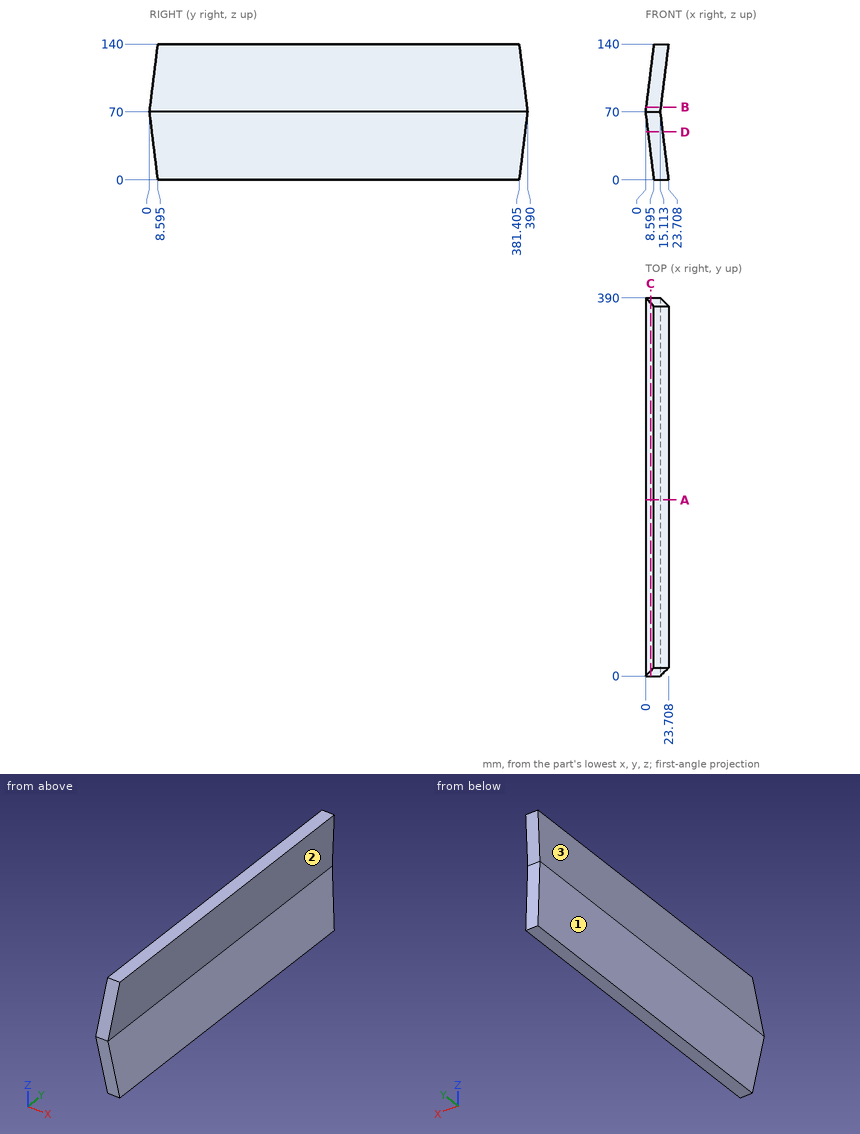
Input: dimensioned drawing with shaded views. Units: mm. Origin: part minimum x, y, z. Coordinates: 2 decimals unless noted, no trailing zeros. Loops run counter-clockwise (first coordinate to the right, second up) from the corner with the lowest first, then second, coordinate; pieces in that order, holes last. Notation, with made-up numbers: M 76.5,-10 L 112.5,-10 A28 cw 112.5,15 Z; hole C 72.5,87 d7. An arc over 180 degrees is marked long. One line per item, written item: value.
(1) Line query: line 1 along X through (y, z) = (51, 6.5); line 2 along X through (y, z) = (159.5, 59.5); line 3 along Y through (x, z) = (3, 87). Output: solid intervals per line, ascending. Write a range as from..to.
Filled in:
line 1: 7.8..22.91
line 2: 1.29..16.4
line 3: 2.09..387.91
(2) Section B-B (z = 75). Output: boundary loops of the cut face in (x, y).
Filled in:
outline: M 0.61,0.61 L 15.73,0.61 L 15.73,389.39 L 0.61,389.39 Z
(3) Section D-D (z = 49.5). Output: boundary loops of the cut face in (x, y), and give its area (3 significant figures).
Filled in:
outline: M 2.52,2.52 L 17.63,2.52 L 17.63,387.48 L 2.52,387.48 Z
area: 5,820 mm^2
(4) Section A-A (y = 181.5). Output: boundary loops of the cut face in (x, z) (1 decimal), and give its area (3 significant figures).
Filled in:
outline: M 0,70 L 8.6,0 L 23.7,0 L 15.1,70 L 23.7,140 L 8.6,140 Z
area: 2,120 mm^2
(5) Pin query (flat end, axial travel): pin 1 (10 mm diameter, centred on y = 171.5, z = 46, fed in from -X); pin 2 (6 mm diameter, centred on x = 13, z = 55.5, fed in from -Y); pin 3 (6 mm diameter, centred on x = 5, z = 78.5, fed in from -Y) (1 decimal). Return the tip coordinate at first contact, or that it passes through.
Filled in:
pin 1: x = 2.33
pin 2: y = 1.41
pin 3: y = 0.7
(6) Pull-direction query (Z, two-part tool) for the marked faces 1, 2 and 3; classes: +Z half, -Z half, draft (parallel to the pull), parting line (faces both ways), or undercut.
Filled in:
face 1: -Z half
face 2: undercut
face 3: +Z half
(7) Section C-C (x = 5.25). Output: boundary loops of the cut face in (y, z).
Filled in:
outline: M 0,70 L 5.25,27.24 L 384.75,27.24 L 390,70 L 384.75,112.76 L 5.25,112.76 Z
